from build123d import *

# Parameters (mm, degrees)
ESQUISSE1_W             = 450
ESQUISSE1_H             = 25
EXTRUSION1_DEPTH        = 10
PLIAGE_START            = -12.5
PLIAGE_1_DEPTH          = 25
PLIAGE_1_2_DEPTH        = 25
ESQUISSE5_R             = 3
ENL_V_MAT_EXTRU_1_DEPTH = 330.361564282
ESQUISSE7_R             = 2.5
ENL_V_MAT_EXTRU_2_DEPTH = 331.27116136


# Read off the part's stored shape, not the designer's step: Pliage 1
with BuildPart() as part:
    # Esquisse1 → Extrusion1 (new body)
    with BuildSketch(Plane.XY):
        with Locations((-225, 0)):
            Rectangle(ESQUISSE1_W, ESQUISSE1_H)
    extrude(amount=EXTRUSION1_DEPTH)

    # Pliage 1 outline → Pliage 1 (cut)
    with BuildSketch(Plane(origin=(0, 0, 0), x_dir=(1, 0, 0), z_dir=(0, 1, 0)).offset(PLIAGE_START)):
        with BuildLine():
            Line((-450, -10), (-238.968577392, -10))
            ThreePointArc((-238.968577392, -10), (-226.653199905, -2.583426132), (-212.511064281, 0))
            Line((-212.511064281, 0), (-450, 0))
            Line((-450, 0), (-450, -10))
        make_face()
    extrude(amount=PLIAGE_1_DEPTH, mode=Mode.SUBTRACT)

    # Pliage 1 2 outline → Pliage 1 2 (add)
    with BuildSketch(Plane(origin=(0, 0, 0), x_dir=(1, 0, 0), z_dir=(0, 1, 0)).offset(PLIAGE_START)):
        with BuildLine():
            ThreePointArc((-238.968577392, -10), (-248.968577392, -23.542486889), (-252.511064281, -40))
            Line((-252.511064281, -40), (-252.511064281, -222.511064281))
            Line((-252.511064281, -222.511064281), (-242.511064281, -222.511064281))
            Line((-242.511064281, -222.511064281), (-242.511064281, -40))
            ThreePointArc((-242.511064281, -40), (-233.724267717, -18.786796564), (-212.511064281, -10))
            Line((-212.511064281, -10), (-238.968577392, -10))
        make_face()
    extrude(amount=PLIAGE_1_2_DEPTH)

    # Esquisse5 → Enlèv. mat.-Extru.1 (cut, through all)
    with BuildSketch(Plane(origin=(-242.511064281, 0, 0), x_dir=(0, 0, -1), z_dir=(1, 0, 0))):
        with Locations((-185, 0)):
            Circle(ESQUISSE5_R)
        with Locations((-60, 0)):
            Circle(ESQUISSE5_R)
    extrude(amount=-ENL_V_MAT_EXTRU_1_DEPTH, mode=Mode.SUBTRACT)

    # Esquisse7 → Enlèv. mat.-Extru.2 (cut, through all)
    with BuildSketch(Plane.XY.offset(10)):
        with Locations((-25, 0)):
            Circle(ESQUISSE7_R)
    extrude(amount=-ENL_V_MAT_EXTRU_2_DEPTH, mode=Mode.SUBTRACT)


solid = part.part
Can you work these out from the model? Positions are in its coordinate system, mm. A direction names the side the tool comes from. Coordinates: 2 decimals unless noted, no trailing zeros. Loops run counter-clockwise (first coordinate to the right, second up) from the corner with the lowest first, then second, coordinate; pieces in that order, holes last. Notation, with made-up numbers: (-14, 2.5) - (27, 2.5) arc R16 ccw to (27, 22.5) - close; hole circle Ø10 at (89.5, -7.75). An arc over 180 degrees is marked (long way). Put each result on its own line as item: value. Start each with the question number.
Item 1: For pin 1 (7.5 mm diameter, centred on x = -96.5, y = 4, fed in from +Z); pin 2 (5.5 mm diameter, centred on y = 0, z = 60, fed in from -X); pin 3 (12.5 mm diameter, centred on y = -3, z = 101, fed in from +X), each with a flat end and sliding along its axis, tell me the tip position at first contact or that it passes through.
Item 2: If I drill on line 1 along Y through (x, z) = (-25, 5); line 2 along Y through (x, z) = (-247, 60); line 3 along Z through (x, y) = (-128, 6.25), over which ranges is the centre line in solid material (lowest first)?
Item 3: Suppose I cut it at B-B (y = 8.5). Please give me the cut outline in (x, z), and give its area (3 significant figures).
Item 4: Suppose I cut it at D-D (z = 140.5). Please give me the cut outline in (x, y), and give its area (3 significant figures).
Item 5: Suppose I cut it at A-A (z = 60). Please give me the cut outline in (x, y), and give its area (3 significant figures).
Item 6: Suppose I cut it at C-C (x = -54.5). Please give me the cut outline in (y, z), and give its area (3 significant figures).
Item 7: If we mould it in two halves opening along Y, with no side actions, what happens to faces 1 (the face through (-247.44, 0.9, 182.14)), 2 (the face through (-183, -12.5, 4)), 3 (the face through (-233.956, -0.175, 19.021))? For each: +Y half, -Y half, draft (parallel to the pull), parting line (faces both ways), or undercut.
Item 8: Which directions (+Z, -Z, +X, -X, +Y, -Y) give clear straight access to the entire face, cutting with the end or side of a thin tool? Please do faces 4 (the face through (-242.511, 0, 133)), 5 (the face through (-248, 0, 222.511)).
Here are the results:
1. pin 1: z = 10
1. pin 2: through
1. pin 3: x = -242.51
2. line 1: -12.5 to -2.5, 2.5 to 12.5
2. line 2: -12.5 to -3, 3 to 12.5
2. line 3: 0 to 10
3. outline: (-252.51, 40) arc R40 ccw to (-212.51, 0) - (0, 0) - (0, 10) - (-212.51, 10) arc R30 cw to (-242.51, 40) - (-242.51, 222.51) - (-252.51, 222.51) - close
3. area: 4,500 mm²
4. outline: (-252.51, -12.5) - (-242.51, -12.5) - (-242.51, 12.5) - (-252.51, 12.5) - close
4. area: 250 mm²
5. outline: (-252.51, -12.5) - (-242.51, -12.5) - (-242.51, -3) - (-252.51, -3) - close; (-252.51, 3) - (-242.51, 3) - (-242.51, 12.5) - (-252.51, 12.5) - close
5. area: 190 mm²
6. outline: (-12.5, 0) - (12.5, 0) - (12.5, 10) - (-12.5, 10) - close
6. area: 250 mm²
7. face 1: undercut
7. face 2: -Y half
7. face 3: draft
8. face 4: +Z, +X, +Y, -Y
8. face 5: +Z, +X, -X, +Y, -Y
